Geometry check sheet. Reference: the model listing, model coordinates, mm. Face numbers are marked on the shaded views. A direction names the side the tool comes from. Round coordinates to 2 decimals unless told otherwise and drop trailing zeros. Write each loop counter-clockwise with the first axis right and the second up, starting at its lowest first coordinate (ties: lowest second). Pieces come first, ordered by that corner, then holes. Notation, with made-up numbers: M -5.5,-19.5 L 37.5,-19.5 A9 ccw 37.5,-2.5 Z; hole C -37,29 d11. An arc over 180 degrees is marked long. Use a Markdown table: item, result.
```python
from build123d import *
from OCP.BRepFilletAPI import BRepFilletAPI_MakeChamfer

# Parameters (mm, degrees)
SKETCH1_W           = 41
SKETCH1_H           = 20
BOSS_EXTRUDE1_DEPTH = 6
CHAMFER1_SIZE       = 3
CHAMFER1_SIZE2      = 1.595128295
BOSS_EXTRUDE2_DEPTH = 5
BOSS_EXTRUDE2_TAPER = 3
SKETCH3_R           = 0.5
BOSS_EXTRUDE3_DEPTH = 5
CUT_EXTRUDE3_DEPTH  = 1.5
SKETCH5_R           = 0.85
CUT_EXTRUDE4_DEPTH  = 55.965898527
FILLET1_R           = 0.5


with BuildPart() as part:
    # Sketch1 → Boss-Extrude1 (new body)
    with BuildSketch(Plane(origin=(0, 0, 0), x_dir=(1, 0, 0), z_dir=(0, 1, 0))):
        with Locations((20.5, 10)):
            Rectangle(SKETCH1_W, SKETCH1_H)
    extrude(amount=BOSS_EXTRUDE1_DEPTH)

    # Chamfer1: one chamfer whose edges measure the first distance from different faces: ONE call of the kernel's chamfer builder (chamfer() names one face for all edges)
    chamfer1_edges_1 = [part.edges().sort_by_distance(p)[0] for p in [
        (41, 6, -10),
    ]]
    chamfer1_side_1 = [part.faces().sort_by_distance(p)[0] for p in [
        (41, 3, -10),
    ]]
    chamfer1_edges_2 = [part.edges().sort_by_distance(p)[0] for p in [
        (20.5, 6, -20),
    ]]
    chamfer1_side_2 = [part.faces().sort_by_distance(p)[0] for p in [
        (20.5, 3, -20),
    ]]
    chamfer1_edges_3 = [part.edges().sort_by_distance(p)[0] for p in [
        (0, 6, -10),
    ]]
    chamfer1_side_3 = [part.faces().sort_by_distance(p)[0] for p in [
        (0, 3, -10),
    ]]
    chamfer1_edges_4 = [part.edges().sort_by_distance(p)[0] for p in [
        (20.5, 6, 0),
    ]]
    chamfer1_side_4 = [part.faces().sort_by_distance(p)[0] for p in [
        (20.5, 3, 0),
    ]]
    chamfer1 = BRepFilletAPI_MakeChamfer(part.part.solid().wrapped)
    for e in chamfer1_edges_1:
        chamfer1.Add(CHAMFER1_SIZE, CHAMFER1_SIZE2, e.wrapped, chamfer1_side_1[0].wrapped)  # the first distance lies on this face
    for e in chamfer1_edges_2:
        chamfer1.Add(CHAMFER1_SIZE, CHAMFER1_SIZE2, e.wrapped, chamfer1_side_2[0].wrapped)  # the first distance lies on this face
    for e in chamfer1_edges_3:
        chamfer1.Add(CHAMFER1_SIZE, CHAMFER1_SIZE2, e.wrapped, chamfer1_side_3[0].wrapped)  # the first distance lies on this face
    for e in chamfer1_edges_4:
        chamfer1.Add(CHAMFER1_SIZE, CHAMFER1_SIZE2, e.wrapped, chamfer1_side_4[0].wrapped)  # the first distance lies on this face
    add(Compound.cast(chamfer1.Shape()), mode=Mode.REPLACE)

    # Sketch2 → Boss-Extrude2 (add)
    with BuildSketch(Plane(origin=(41, 0, 0), x_dir=(0, 0, -1), z_dir=(1, 0, 0))):
        Polygon((10, 2), (7.5, 2), (7.5, 0), (12.260148274, 0), (12.260148274, 2), align=None)
    extrude(amount=BOSS_EXTRUDE2_DEPTH, taper=BOSS_EXTRUDE2_TAPER)

    # Sketch3 → Boss-Extrude3 (add)
    with BuildSketch(Plane(origin=(46, 0, 0), x_dir=(0, 0, -1), z_dir=(1, 0, 0))):
        with Locations((8.5, 1)):
            Circle(SKETCH3_R)
        with Locations((9.8, 1)):
            Circle(SKETCH3_R)
        with Locations((11.1, 1)):
            Circle(SKETCH3_R)
    extrude(amount=BOSS_EXTRUDE3_DEPTH)

    # Sketch4 → Cut-Extrude3 (cut)
    with BuildSketch(Plane(origin=(0, 6, 0), x_dir=(1, 0, 0), z_dir=(0, 1, 0))):
        with BuildLine():
            Line((38.697764924, 0.652235076), (37.047764924, 0.652235076))
            Line((37.047764924, 0.652235076), (37.047764924, 2.302235076))
            ThreePointArc((37.047764924, 2.302235076), (37.531038735, 3.468961265), (38.697764924, 3.952235076))
            Line((38.697764924, 3.952235076), (40.347764924, 3.952235076))
            Line((40.347764924, 3.952235076), (40.347764924, 2.302235076))
            Line((40.347764924, 2.302235076), (40.347764924, 0.652235076))
            Line((40.347764924, 0.652235076), (38.697764924, 0.652235076))
        make_face()
        with BuildLine():
            Line((37.047764924, 17.697764924), (37.047764924, 19.347764924))
            Line((37.047764924, 19.347764924), (38.697764924, 19.347764924))
            Line((38.697764924, 19.347764924), (40.347764924, 19.347764924))
            Line((40.347764924, 19.347764924), (40.347764924, 17.697764924))
            Line((40.347764924, 17.697764924), (40.347764924, 16.047764924))
            Line((40.347764924, 16.047764924), (38.697764924, 16.047764924))
            ThreePointArc((38.697764924, 16.047764924), (37.531038735, 16.531038735), (37.047764924, 17.697764924))
        make_face()
        with BuildLine():
            Line((2.302235076, 16.047764924), (0.652235076, 16.047764924))
            Line((0.652235076, 16.047764924), (0.652235076, 17.697764924))
            Line((0.652235076, 17.697764924), (0.652235076, 19.347764924))
            Line((0.652235076, 19.347764924), (2.302235076, 19.347764924))
            Line((2.302235076, 19.347764924), (3.952235076, 19.347764924))
            Line((3.952235076, 19.347764924), (3.952235076, 17.697764924))
            ThreePointArc((3.952235076, 17.697764924), (3.468961265, 16.531038735), (2.302235076, 16.047764924))
        make_face()
        with BuildLine():
            Line((3.952235076, 2.302235076), (3.952235076, 0.652235076))
            Line((3.952235076, 0.652235076), (2.302235076, 0.652235076))
            Line((2.302235076, 0.652235076), (0.652235076, 0.652235076))
            Line((0.652235076, 0.652235076), (0.652235076, 2.302235076))
            Line((0.652235076, 2.302235076), (0.652235076, 3.952235076))
            Line((0.652235076, 3.952235076), (2.302235076, 3.952235076))
            ThreePointArc((2.302235076, 3.952235076), (3.468961265, 3.468961265), (3.952235076, 2.302235076))
        make_face()
    extrude(amount=-CUT_EXTRUDE3_DEPTH, mode=Mode.SUBTRACT)

    # Sketch5 → Cut-Extrude4 (cut, through all)
    with BuildSketch(Plane(origin=(0, 4.5, 0), x_dir=(1, 0, 0), z_dir=(0, 1, 0))):
        with Locations(Location((38.625100388, 2.374899612, 0), (0, 0, 270))):
            Circle(SKETCH5_R)
        with Locations(Location((38.625100388, 17.625100388, 0), (0, 0, 270))):
            Circle(SKETCH5_R)
        with Locations(Location((2.374899612, 17.625100388, 0), (0, 0, 270))):
            Circle(SKETCH5_R)
        with Locations(Location((2.374899612, 2.374899612, 0), (0, 0, 270))):
            Circle(SKETCH5_R)
    extrude(amount=-CUT_EXTRUDE4_DEPTH, mode=Mode.SUBTRACT)

    # Fillet1
    # the kernel refuses this fillet: 0.5 mm, written as the material it takes off along each edge
    with BuildSketch(Plane(origin=(-0.424571433, 2.20149727, -20.424571433), x_dir=(-0.19951100260176627, -0.3752256227209219, 0.9052077617290598), z_dir=(0.42496930254486104, 0.79925101425589, 0.42496930254486104)), Plane(origin=(-0.424571433, 2.20149727, 0.424571433), x_dir=(0.9052077617290598, -0.3752256227209218, 0.19951100260176646), z_dir=(0.42496930254486104, 0.79925101425589, -0.42496930254486104))) as fillet1_piece_1:
        with BuildLine():
            CenterArc((FILLET1_R * 0.799251014256, FILLET1_R), FILLET1_R, 192.732736423, 77.267263577)
            Line((-FILLET1_R * 0.176157759496, FILLET1_R * 0.779596451735), (0, 0))
            Line((0, 0), (FILLET1_R * 0.799251014256, 0))
        make_face()
    extrude(amount=3.874884616, mode=Mode.SUBTRACT)
    with BuildSketch(Plane(origin=(0, -1.25, -20), x_dir=(0, 0, 1), z_dir=(0, 1, 0)), Plane(origin=(0, -1.25, 0), x_dir=(1, 0, 0), z_dir=(0, 1, 0))) as fillet1_piece_2:
        with BuildLine():
            CenterArc((FILLET1_R, FILLET1_R), FILLET1_R, 180, 90)
            Line((0, FILLET1_R), (0, 0))
            Line((0, 0), (FILLET1_R, 0))
        make_face()
    extrude(amount=5.5, mode=Mode.SUBTRACT)
    with BuildSketch(Plane(origin=(41.424571433, 2.20149727, 0.424571433), x_dir=(-0.9052077617290598, -0.37522562272092175, 0.1995110026017665), z_dir=(-0.42496930254486104, 0.79925101425589, -0.42496930254486104)), Plane(origin=(41.424571433, 2.20149727, -20.424571433), x_dir=(0.1995110026017654, -0.37522562272092236, 0.9052077617290599), z_dir=(-0.42496930254486104, 0.79925101425589, 0.42496930254486104))) as fillet1_piece_3:
        with BuildLine():
            CenterArc((FILLET1_R * 0.799251014256, -FILLET1_R), FILLET1_R, 90, 77.267263577)
            Line((-FILLET1_R * 0.176157759496, -FILLET1_R * 0.779596451735), (0, 0))
            Line((0, 0), (FILLET1_R * 0.799251014256, 0))
        make_face()
    extrude(amount=3.874884616, mode=Mode.SUBTRACT)
    with BuildSketch(Plane(origin=(41, -1.25, -20), x_dir=(0, 0, 1), z_dir=(0, 1, 0)), Plane(origin=(41, -1.25, 0), x_dir=(-1, 0, 0), z_dir=(0, 1, 0))) as fillet1_piece_4:
        with BuildLine():
            CenterArc((FILLET1_R, -FILLET1_R), FILLET1_R, 90, 90)
            Line((0, -FILLET1_R), (0, 0))
            Line((0, 0), (FILLET1_R, 0))
        make_face()
    extrude(amount=5.5, mode=Mode.SUBTRACT)


solid = part.part
```
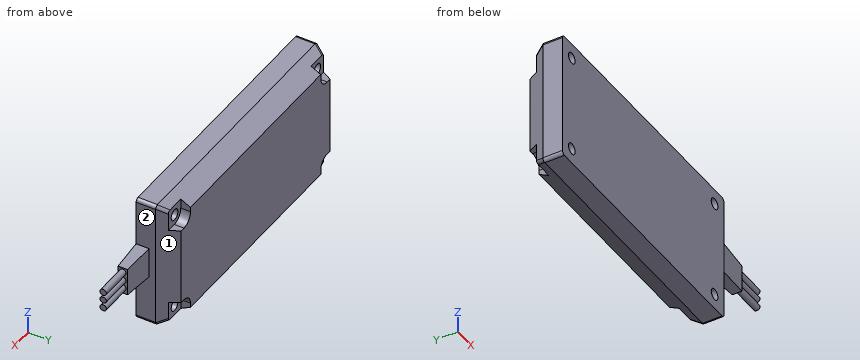
Item 1: Cross-section at A-A, the plane x = 35.5. Record the cut outline in (y, z), and give its area (3 significant figures).
Outcome:
| item | result |
|---|---|
| outline | M 0,-20 L 3,-20 L 6,-18.4 L 6,-1.6 L 3,0 L 0,0 Z |
| area | 115 mm2 |
Item 2: Go/stop test with flat-tipped pins: pin 1 (1.2 mm diameter, centred on x = 39.5, y = 5.5, fed in from +Z); pin 2 (1.2 mm diameter, centred on y = 5, z = -18.5, fed in from +X); pin 3 (0.9 mm diameter, centred on x = 1.5, z = -2.5, fed in from +Y). Record where each tip stops, or that it passes through.
Outcome:
| item | result |
|---|---|
| pin 1 | stops at z = -3.95 |
| pin 2 | stops at x = 40.26 |
| pin 3 | stops at y = 4.5 |
Item 3: Access from +Z, -Z, +X, -X, +Y, -Y to the whole of each face (thin tool, end or side, straight path). Record for the marked faces 1 and 2.
Outcome:
| item | result |
|---|---|
| face 1 | +Z, -Z, +X, +Y |
| face 2 | +X, +Y |
Item 4: Material ranges on line 1 along Z through (x, y) = (21.5, 4.5); line 2 along X through (y, z) = (2, -2); line 3 along X through (y, z) = (1.5, -15), recorded low to high. Write a range as from..to.
Outcome:
| item | result |
|---|---|
| line 1 | z = -19.2..-0.8 |
| line 2 | x = 0..1.61, 3.14..37.86, 39.39..41 |
| line 3 | x = 0..41 |
Item 5: Cross-section at D-D, the plane y = 1. Count the separate pieces of the cut face and the enclosed holes in it, and give its area (3 significant figures).
Outcome:
| item | result |
|---|---|
| separate pieces | 1 |
| enclosed holes | 4 |
| area | 848 mm2 |
Item 6: Cross-section at B-B, the plane z = -5.5. Record the cut outline in (x, y), and give its area (3 significant figures).
Outcome:
| item | result |
|---|---|
| outline | M 0,0 L 41,0 L 41,3 L 39.4,6 L 1.6,6 L 0,3 Z |
| area | 241 mm2 |
Item 7: Cross-section at C-C, the plane y = 5.25. Record the cut outline in (x, z).
Outcome:
| item | result |
|---|---|
| outline | M 1.2,-16.05 L 2.3,-16.05 A1.65 cw 3.95,-17.7 L 3.95,-18.8 L 37.05,-18.8 L 37.05,-17.7 A1.65 cw 38.7,-16.05 L 39.8,-16.05 L 39.8,-3.95 L 38.7,-3.95 A1.65 cw 37.05,-2.3 L 37.05,-1.2 L 3.95,-1.2 L 3.95,-2.3 A1.65 cw 2.3,-3.95 L 1.2,-3.95 Z |
